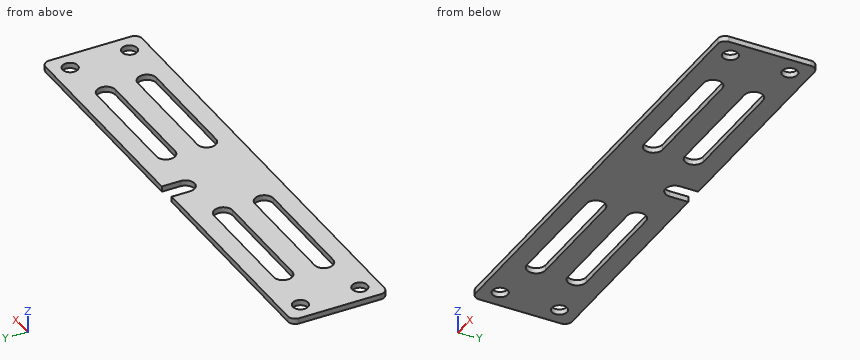
from build123d import *

# Parameters (mm, degrees)
SKETCH_1_W          = 126
SKETCH_1_H          = 26
EXTRUDE_1_DEPTH     = 1.5
FILLET_1_R          = 2
SKETCH_2_W          = 5
SKETCH_2_H          = 15
CUT_EXTRUDE_1_DEPTH = 65.344774458
FILLET_2_R          = 2.5
CUT_EXTRUDE_2_DEPTH = 65.344774458
SKETCH_4_R          = 2.05
CUT_EXTRUDE_3_DEPTH = 65.344774458


with BuildPart() as part:
    # 草图1 → 凸台-拉伸1 (new body)
    with BuildSketch(Plane.XY):
        Rectangle(SKETCH_1_W, SKETCH_1_H)
    extrude(amount=EXTRUDE_1_DEPTH)

    # 圆角1
    fillet_1_edges = [part.edges().sort_by_distance(p)[0] for p in [
        (-63, 13, 0.75),
        (63, 13, 0.75),
        (63, -13, 0.75),
        (-63, -13, 0.75),
    ]]
    fillet(fillet_1_edges, radius=FILLET_1_R)

    # 草图2 → 切除-拉伸1 (cut, through all)
    with BuildSketch(Plane.XY.offset(1.5)):
        with Locations((0, 13)):
            Rectangle(SKETCH_2_W, SKETCH_2_H)
    extrude(amount=-CUT_EXTRUDE_1_DEPTH, mode=Mode.SUBTRACT)

    # 圆角2
    fillet_2_edges = [part.edges().sort_by_distance(p)[0] for p in [
        (2.5, 5.5, 0.75),
        (-2.5, 5.5, 0.75),
    ]]
    fillet(fillet_2_edges, radius=FILLET_2_R - 0.0001)  # a hair under: the kernel refuses the full size

    # 草图3 → 切除-拉伸2 (cut, through all)
    with BuildSketch(Plane.XY.offset(1.5)):
        with BuildLine():
            Line((-44.5, 8), (-14.5, 8))
            ThreePointArc((-14.5, 8), (-12, 5.5), (-14.5, 3))
            Line((-14.5, 3), (-44.5, 3))
            ThreePointArc((-44.5, 3), (-47, 5.5), (-44.5, 8))
        make_face()
        with BuildLine():
            Line((14.5, 8), (44.5, 8))
            ThreePointArc((44.5, 8), (47, 5.5), (44.5, 3))
            Line((44.5, 3), (14.5, 3))
            ThreePointArc((14.5, 3), (12, 5.5), (14.5, 8))
        make_face()
        with BuildLine():
            Line((14.5, -3), (44.5, -3))
            ThreePointArc((44.5, -3), (47, -5.5), (44.5, -8))
            Line((44.5, -8), (14.5, -8))
            ThreePointArc((14.5, -8), (12, -5.5), (14.5, -3))
        make_face()
        with BuildLine():
            Line((-44.5, -3), (-14.5, -3))
            ThreePointArc((-14.5, -3), (-12, -5.5), (-14.5, -8))
            Line((-14.5, -8), (-44.5, -8))
            ThreePointArc((-44.5, -8), (-47, -5.5), (-44.5, -3))
        make_face()
    extrude(amount=-CUT_EXTRUDE_2_DEPTH, mode=Mode.SUBTRACT)

    # 草图4 → 切除-拉伸3 (cut, through all)
    with BuildSketch(Plane.XY.offset(1.5)):
        with Locations((58, -8)):
            Circle(SKETCH_4_R)
        with Locations((58, 8)):
            Circle(SKETCH_4_R)
        with Locations((-58, 8)):
            Circle(SKETCH_4_R)
        with Locations((-58, -8)):
            Circle(SKETCH_4_R)
    extrude(amount=-CUT_EXTRUDE_3_DEPTH, mode=Mode.SUBTRACT)


solid = part.part
Input: part model. Units: mm. Frame: model coordinates. Give positions to 0.01 mm unless a question says otherwise; leave off trailing zeros. Loops run counter-clockwise (first coordinate to the right, second up) from the corner with the lowest first, then second, coordinate; pieces in that order, holes last. Notation, with made-up numbers: M 46.25,49.25 L 97.25,49.25 A26 cw 97.25,88.25 Z; hole C -2,-10.75 d3. An arc over 180 degrees is marked long. Use one line per item in the form item = value.
1. Line query: L1, parallel to Y at x = 58, z = 0.7; L2, parallel to Y at x = -43.5, z = 0.5; L3, parallel to X at y = 11, z = 0.5. Output: solid intervals per line, ascending.
Numbers:
L1 = -13 to -10.05, -5.95 to 5.95, 10.05 to 13
L2 = -13 to -8, -3 to 3, 8 to 13
L3 = -63 to -2.5, 2.5 to 63
2. Section query A-A, the plane x = -58. Return the cut outline in (y, z).
Numbers:
outline = M -13,0 L -10.05,0 L -10.05,1.5 L -13,1.5 Z; M -5.95,0 L 5.95,0 L 5.95,1.5 L -5.95,1.5 Z; M 10.05,0 L 13,0 L 13,1.5 L 10.05,1.5 Z
3. Section query C-C, the plane x = 25.5. Return the cut outline in (y, z), and give its area (3 significant figures).
Numbers:
outline = M -13,0 L -8,0 L -8,1.5 L -13,1.5 Z; M -3,0 L 3,0 L 3,1.5 L -3,1.5 Z; M 8,0 L 13,0 L 13,1.5 L 8,1.5 Z
area = 24.0 mm²
4. Section query B-B, the plane z = 0.55. Count the separate pieces of the cut face and the enclosed holes in it, and give its area (3 significant figures).
Numbers:
separate_pieces = 1
enclosed_holes = 8
area = 2,510 mm²
5. First-contact query: pin 1 (10 mm diameter, centred on x = 22.5, y = 8, fed in from -Z). Flat tip, straight axial feed; report the tip coordinate or a pass-through.
Numbers:
pin_1 = 0
